The model under review builds one solid part; all positions refer to its coordinate system, in mm. A direction names the side the tool comes from. Give positions to 0.01 mm unless a question says otherwise; leave off trailing zeros. Order: outer loops, then holes, each group sorted by start corner. A loop starts at its lowest first (then second) coordinate and runs counter-clockwise, first axis right, second up.
```python
from build123d import *

# Parameters (mm, degrees)
F0_R     = 280
F1_DEPTH = 16
F2_R     = 30
F2_R_2   = 4.5
F3_DEPTH = 25
F4_R     = 44.25
F4_R_2   = 4.5
F4_R_3   = 30
F5_DEPTH = 3


# Not quite as in the source:
# - a feature names something its author has since deleted; it is built from what else it names


with BuildPart() as f1:
    # F0 (on Top) → F1 (new body)
    with BuildSketch(Plane.XY):
        Circle(F0_R)
    extrude(amount=F1_DEPTH)

    # F2 (on face) → F3 (cut)
    with BuildSketch(Plane.XY.offset(16)):
        Circle(F2_R)
        with Locations((-37.25, 0)):
            Circle(F2_R_2)
        with Locations((0, 37.25)):
            Circle(F2_R_2)
        with Locations((37.25, 0)):
            Circle(F2_R_2)
        with Locations((0, -37.25)):
            Circle(F2_R_2)
    extrude(amount=-F3_DEPTH, mode=Mode.SUBTRACT)

    # F4 (on face) → F5 (cut)
    with BuildSketch(Plane(origin=(0, 0, 0), x_dir=(1, 0, 0), z_dir=(0, 0, -1))):
        Circle(F4_R)
        with Locations((0, -37.25)):
            Circle(F4_R_2, mode=Mode.SUBTRACT)
        with Locations((-37.25, 0)):
            Circle(F4_R_2, mode=Mode.SUBTRACT)
        Circle(F4_R_3, mode=Mode.SUBTRACT)
        with Locations((37.25, 0)):
            Circle(F4_R_2, mode=Mode.SUBTRACT)
        with Locations((0, 37.25)):
            Circle(F4_R_2, mode=Mode.SUBTRACT)
    extrude(amount=-F5_DEPTH, mode=Mode.SUBTRACT)


solid = f1.part
```
1. Take a section at B-B (x = 132). Write out the cut boundary in (y, z), and give its area (3 significant figures).
2. Insertion check: pin 1 (11.5 mm diameter, centred on x = 0, y = 37.25, fed in from -Z); pin 2 (4 mm diameter, centred on y = 124, z = 13, fed in from +X); pin 3 (4 mm diameter, centred on y = -115, z = 3, fed in from +X). Each pin has a flat end and moves straight along its axis. Give the tip position at first contact, or say it passes through.
3. Draft analysis for pull direction X (two halves, no side actions). For faces 3 (the cylindrical face through (-9.59, 43.2, 1.48)), 4 (the cylindrical face through (-29.97, 1.32, 9.59)), 5 (the cylindrical face through (-222.198, -170.376, 7.888)), 6 (the flat face through (-4, -58, 0)), state which applies: pulls with the +X half, pulls with the -X half, needs draft (parallel to the pull), parting line crosses it, or undercut.
4. Take a section at A-A (y = 224). Write out the cut boundary in (x, z), and give its area (3 significant figures).
5. For faces 1 (the flat face through (29, 9, 3)), 2 (the flat face through (-4, -58, 16)), list the 3-axis set-ups (+Z, -Z, +X, -X, +Y, -Y) from which the entire face can be reached by the end or side of a thin tool; tool diameter is ignored.
6. To check wall thickness, follow line 1 (Y direction, x = 0, z = 9.25); line 2 (Y direction, x = -34.5, z = 1); line 3 (X direction, y = -37.25, z = 7). State the ranges of each line that lie inside material, in increasing order.
Answer:
1. outline: (-246.93, 0) - (246.93, 0) - (246.93, 16) - (-246.93, 16) - close
1. area: 7,900 mm2
2. pin 1: stops at z = 3
2. pin 2: stops at x = 252.02
2. pin 3: stops at x = 256.19
3. face 3: undercut
3. face 4: undercut
3. face 5: parting line crosses it
3. face 6: needs draft
4. outline: (-168, 0) - (168, 0) - (168, 16) - (-168, 16) - close
4. area: 5,380 mm2
5. face 1: -Z
5. face 2: +Z, +X, -X, +Y, -Y
6. line 1: y = -280 to -41.75, -32.75 to -30, 30 to 32.75, 41.75 to 280
6. line 2: y = -277.87 to -27.71, 27.71 to 277.87
6. line 3: x = -277.51 to -4.5, 4.5 to 277.51
